Check sheet for the modelled part. Datum: model origin and axes. Units: mm. A direction names the side the tool comes from. Coordinates: 2 decimals unless noted, no trailing zeros. Write each loop counter-clockwise with the first axis right and the second up, starting at its lowest first coordinate (ties: lowest second). Pieces come first, ordered by that corner, then holes. Notation, with made-up numbers: M -12,54.5 L 37,54.5 A22 ccw 37,78.5 Z; hole C -31,-6.5 d7. An arc over 180 degrees is marked long. Answer as CSV lines item,"result". Start each with the question number.
Q1. Sectioned sample at C-C, the plane z = -6. Record the cut outline in (x, y), then the cut area to 3 significant figures.
Q2. Depth check by flat-ended pin: pin 1 Ø4 at (x, z) = (15.5, 18.5) entering from +Y; pin 2 Ø2 at (x, y) = (5.5, 22) entering from +Z; pin 3 Ø8 at (y, z) = (44, -17.5) entering from +X; pin 4 Ø8 at (x, y) = (21, 6.5) entering from +Z. Enter the tip coordinate at first touch or a pass-through.
Q3. Sectioned sample at D-D, the plane y = 28. Record the cut outline in (x, z).
Q4. Mould release check, pull along Z, two halves, no side actions. Record for faces 4 (the flat face through (-15.14, 39.94, 15.21)), 5 (the flat face through (25, 10, 10)), 6 (the flat face through (20, 10, 5)), 7 (the flat face through (15, 10, -5)): pulls with the +Z half, pulls with the -Z half, needs draft (parallel to the pull), parting line crosses it, or undercut.
Q5. Sectioned sample at B-B, the plane x = -10. Record the cut outline in (y, z).
Q6. Access from +Z, -Z, +X, -X, +Y, -Y to the whole of each face (thin tool, end or side, straight path). Record for faces 1 (the flat face through (20, 10, -15)), 2 (the flat face through (-10, 15, 25)), 3 (the flat face through (-5, 35, -5)).
Q7. Sectioned sample at A-A, the plane y = 17. Record the cut outline in (x, z).
Q8. Thickness scan on line 1 along X through (y, z) = (20.5, 17.5); line 2 along X through (y, z) = (9.5, -11.5); line 3 along Y through (x, z) = (2.5, 8.5). Record the ranges inside material, lowest first. Write a range as from..to.
from build123d import *

# Parameters (mm, degrees)
SKETCH1_W               = 50
SKETCH1_H               = 50
BOSS_EXTRUDE1_DEPTH     = 50
CUT_EXTRUDE2_DEPTH      = 76
SKETCH4_W               = 20
SKETCH4_H               = 20
CUT_EXTRUDE3_DEPTH      = 10
CUT_EXTRUDE4_DEPTH      = 64.442887702
CUT_EXTRUDE4_DEPTH_BACK = 64.442887702
CUT_EXTRUDE5_DEPTH      = 47.368092477
CUT_EXTRUDE5_DEPTH_BACK = 47.368092477


with BuildPart() as part:
    # Sketch1 → Boss-Extrude1 (new body)
    with BuildSketch(Plane(origin=(0, 0, 0), x_dir=(1, 0, 0), z_dir=(0, 1, 0))):
        Rectangle(SKETCH1_W, SKETCH1_H)
    extrude(amount=BOSS_EXTRUDE1_DEPTH)

    # Sketch3 → Cut-Extrude2 (cut, through all)
    with BuildSketch(Plane.XY.offset(25)):
        Polygon((-5, 50), (-5, 20), (25.055791763, 20), (25, 50), align=None)
    extrude(amount=-CUT_EXTRUDE2_DEPTH, mode=Mode.SUBTRACT)

    # Sketch4 → Cut-Extrude3 (cut)
    with BuildSketch(Plane(origin=(25, 0, 0), x_dir=(0, 0, -1), z_dir=(1, 0, 0))):
        with Locations((5, 10)):
            Rectangle(SKETCH4_W, SKETCH4_H)
    extrude(amount=-CUT_EXTRUDE3_DEPTH, mode=Mode.SUBTRACT)

    # Sketch8 → Cut-Extrude4 (cut, two sides: drawn at the far end of the back side and taken through both)
    with BuildSketch(Plane(origin=(-5, 0, 0), x_dir=(0, 0, -1), z_dir=(1, 0, 0)).offset(-CUT_EXTRUDE4_DEPTH_BACK)):
        Polygon((-114.864472803, -59.71478058), (-25.149692223, 30), (-5, 50.149692223), (84.71478058, 139.864472803), (-94.71478058, 319.294033964), (-294.294033964, 119.71478058), align=None)
    extrude(amount=CUT_EXTRUDE4_DEPTH + CUT_EXTRUDE4_DEPTH_BACK, mode=Mode.SUBTRACT)

    # Sketch9 → Cut-Extrude5 (cut, two sides: drawn at the far end of the back side and taken through both)
    with BuildSketch(Plane(origin=(0, 20, 0), x_dir=(1, 0, 0), z_dir=(0, 1, 0)).offset(-CUT_EXTRUDE5_DEPTH_BACK)):
        Polygon((148.701256003, 46.638963739), (25.059091939, -15), (5, -25), (-118.642164064, -86.638963739), (4.635763413, -333.923291867), (271.97918348, -200.64536439), align=None)
    extrude(amount=CUT_EXTRUDE5_DEPTH + CUT_EXTRUDE5_DEPTH_BACK, mode=Mode.SUBTRACT)


solid = part.part
Output:
1,outline,"M -25,0 L 15,0 L 15,20 L -5,20 L -5,50 L -25,50 Z"
1,area,"1,400 mm^2"
2,pin 1,"stops at y = 20"
2,pin 2,"passes through"
2,pin 3,"stops at x = -5"
2,pin 4,"stops at z = 19.02"
3,outline,"M -25,-25 L -5,-25 L -5,25 L -25,25 Z"
4,face 4,"pulls with the +Z half"
4,face 5,"needs draft"
4,face 6,"undercut"
4,face 7,"undercut"
5,outline,"M 0,-25 L 50,-25 L 50,5.15 L 30.15,25 L 0,25 Z"
6,face 1,"+X, +Y, -Y"
6,face 2,"+Z, +X, -X, +Y, -Y"
6,face 3,"+Z, -Z, +X, +Y"
7,outline,"M -25,-25 L 25,-25 L 25,-15 L 15,-15 L 15,5 L 25,5 L 25,15.03 L 5,25 L -25,25 Z"
8,line 1,"x = -25..-5"
8,line 2,"x = -25..15"
8,line 3,"y = 0..20"
